```python
from build123d import *

# Parameters (mm, degrees)
EXTRUDE_1_DEPTH     = 4.8
SKETCH_2_W          = 5
SKETCH_2_H          = 4.8
SKETCH_2_W_2        = 2
SKETCH_2_H_2        = 23
EXTRUDE_2_DEPTH     = 12
SKETCH_3_R          = 0.95
CUT_EXTRUDE_1_DEPTH = 5
SKETCH_6_R          = 0.95
CUT_EXTRUDE_4_DEPTH = 32
SKETCH_7_W          = 42.8
SKETCH_7_H          = 6
EXTRUDE_3_DEPTH     = 5
SKETCH_8_W          = 4
SKETCH_8_H          = 32.6
EXTRUDE_4_DEPTH     = 3
SKETCH_9_W          = 42.8
SKETCH_9_H          = 12.6
EXTRUDE_6_DEPTH     = 5
SKETCH_11_R         = 0.95
CUT_EXTRUDE_5_DEPTH = 47.323752007
SKETCH_12_W         = 0.5
SKETCH_12_H         = 25.6
CUT_EXTRUDE_6_DEPTH = 0.5


with BuildPart() as part:
    # 草图1 → 凸台-拉伸1 (new body)
    with BuildSketch(Plane.XY):
        Polygon((12, 0), (28.3, 0), (28.3, -23), (12, -23), (12, -27.8), (4.4, -27.8), (4.4, -23), (0, -23), (0, 0), (4.4, 0), (4.4, 4.8), (12, 4.8), align=None)
    extrude(amount=EXTRUDE_1_DEPTH)

    # 草图2 → 凸台-拉伸2 (add)
    with BuildSketch(Plane.XY.offset(4.8)):
        with Locations((9.5, 2.4)):
            Rectangle(SKETCH_2_W, SKETCH_2_H)
        with Locations((9.5, -25.4)):
            Rectangle(SKETCH_2_W, SKETCH_2_H)
        with Locations((27.3, -11.5)):
            Rectangle(SKETCH_2_W_2, SKETCH_2_H_2)
    extrude(amount=EXTRUDE_2_DEPTH)

    # 草图3 → 切除-拉伸1 (cut)
    with BuildSketch(Plane.ZY.offset(-7)):
        with Locations((10.8, 2.4)):
            Circle(SKETCH_3_R)
        with Locations((10.8, -25.4)):
            Circle(SKETCH_3_R)
    extrude(amount=-CUT_EXTRUDE_1_DEPTH, mode=Mode.SUBTRACT)

    # 草图6 → 切除-拉伸4 (cut)
    with BuildSketch(Plane(origin=(0, 0, 0), x_dir=(1, 0, 0), z_dir=(0, 1, 0))):
        with Locations(Location((14, -2.4, 0), (0, 0, 270))):
            Circle(SKETCH_6_R)
    extrude(amount=-CUT_EXTRUDE_4_DEPTH, mode=Mode.SUBTRACT)

    # 草图7 → 凸台-拉伸3 (add)
    with BuildSketch(Plane(origin=(0, 0, 0), x_dir=(-1, 0, 0), z_dir=(0, 0, -1))):
        with Locations((-6.9, -5.2)):
            Rectangle(SKETCH_7_W, SKETCH_7_H)
    extrude(amount=EXTRUDE_3_DEPTH)

    # 草图8 → 凸台-拉伸4 (add)
    with BuildSketch(Plane.XY):
        with Locations((-2, -11.5)):
            Rectangle(SKETCH_8_W, SKETCH_8_H)
        with Locations((-12.5, -11.5)):
            Rectangle(SKETCH_8_W, SKETCH_8_H)
    extrude(amount=EXTRUDE_4_DEPTH)

    # 草图9 → 凸台-拉伸6 (add)
    with BuildSketch(Plane(origin=(0, 0, 0), x_dir=(-1, 0, 0), z_dir=(0, 0, -1))):
        with Locations((-6.9, -21.5)):
            Rectangle(SKETCH_9_W, SKETCH_9_H)
    extrude(amount=EXTRUDE_6_DEPTH)

    # 草图11 → 切除-拉伸5 (cut, through all)
    with BuildSketch(Plane(origin=(0, 4.8, 0), x_dir=(1, 0, 0), z_dir=(0, 1, 0))):
        with Locations(Location((7, -2.4, 0), (0, 0, 180))):
            Circle(SKETCH_11_R)
    extrude(amount=-CUT_EXTRUDE_5_DEPTH, mode=Mode.SUBTRACT)

    # 草图12 → 切除-拉伸6 (cut)
    with BuildSketch(Plane(origin=(0, 0, -5), x_dir=(-1, 0, 0), z_dir=(0, 0, -1))):
        with Locations((-18.05, -15)):
            Rectangle(SKETCH_12_W, SKETCH_12_H)
        with Locations((-0.75, -15)):
            Rectangle(SKETCH_12_W, SKETCH_12_H)
    extrude(amount=-CUT_EXTRUDE_6_DEPTH, mode=Mode.SUBTRACT)


solid = part.part
```
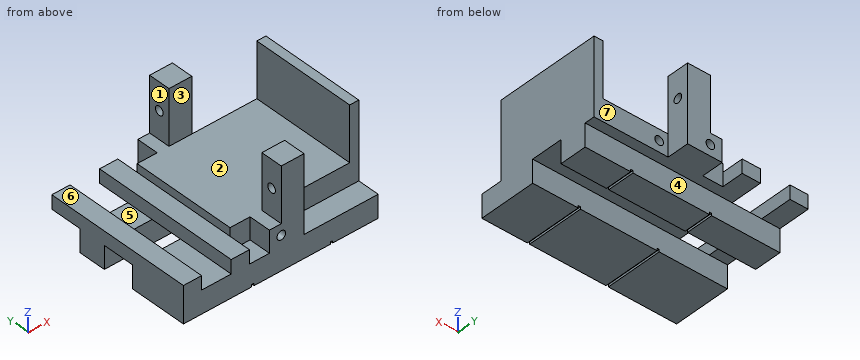
Input: part model. Units: mm. Frame: model coordinates. Face numbers are marked on the shaded views. A direction names the side the tool comes from. Give positions to 0.01 mm unless a question says otherwise; leave off trailing zeros. Write each loop counter-clockwise with the first axis right and the second up, starting at its lowest first coordinate (ties: lowest second). Pieces come first, ordered by that corner, then holes. Notation, with made-up numbers: (54.5, 52.5) - (73.5, 52.5) arc R19 cw to (73.5, 85.5) - close; hole circle Ø9 at (15.25, 44.5). An arc over 180 degrees is marked (long way). Write item = value, one per line. Start each with the question number.
1. Ray query, L1, parallel to Y at x = 9.55, z = 10.8; L2, parallel to Z at x = 7, y = -5; L3, parallel to Z at x = 4, y = -22.5. Return the intervals inside material, ascending.
2. Section query C-C, the plane z = 6.75. Output: boundary loops of the cut face in (x, y), then the cut area to 3 significant figures.
3. First-contact query: pin 1 Ø4 at (x, z) = (15, 1.5) entering from +Y; pin 2 Ø1 at (x, y) = (2, -16.5) entering from +Z; pin 3 Ø2.5 at (y, z) = (3, 9) entering from +X. Flat tips, straight axial feed; report the tip coordinate or a pass-through.
4. Mould query, pull axis Y, two halves, no side actions, for the marked faces 1, 2, 3 and 4. Classes: released by +Y, released by -Y, zero draft, split by the parting line, or undercut.
5. Section query A-A, the plane y = -11. Output: boundary loops of the cut face in (x, z), then the cut area to 3 significant figures.
6. Access query for the marked faces 5, 6 and 7. Directions: +Z, -Z, +X, -X, +Y, -Y. A direction counts if a zero-diameter tool reaches every point of the face in a straight line with its end or side. Return the directions, or none.
7. Section query D-D, the plane y = -25.4. Count the separate pieces of the cut face and the enclosed holes in it, then the cut area to 3 significant figures.
8. Section query B-B, the plane x = 14. Output: boundary loops of the cut face in (y, z).
Check sheet entries:
q1.L1 = -27.8 to -26.35, -24.45 to -23, 0 to 1.45, 3.35 to 4.8
q1.L2 = -5 to 1.45, 3.35 to 4.8
q1.L3 = -5 to 4.8
q2.outline = (7, -27.8) - (12, -27.8) - (12, -23) - (7, -23) - close; (7, 0) - (12, 0) - (12, 4.8) - (7, 4.8) - close; (26.3, -23) - (28.3, -23) - (28.3, 0) - (26.3, 0) - close
q2.area = 94.0 mm2
q3.pin_1 = 0
q3.pin_2 = 4.8
q3.pin_3 = 12
q4.face_1 = zero draft
q4.face_2 = undercut
q4.face_3 = undercut
q4.face_4 = released by +Y
q5.outline = (-14.5, 0) - (-10.5, 0) - (-10.5, 3) - (-14.5, 3) - close; (-4, 0) - (28.3, 0) - (28.3, 16.8) - (26.3, 16.8) - (26.3, 4.8) - (0, 4.8) - (0, 3) - (-4, 3) - close; hole circle Ø1.9 at (7, 2.4); hole circle Ø1.9 at (14, 2.4)
q5.area = 178 mm2
q6.face_5 = +Z, +Y, -Y
q6.face_6 = +Z, -X, +Y, -Y
q6.face_7 = +Z, -Z, +X, +Y
q7.separate_pieces = 2
q7.enclosed_holes = 1
q7.area = 322 mm2
q8.outline = (-27.8, -5) - (-15.2, -5) - (-15.2, 0) - (-8.2, 0) - (-8.2, -5) - (-2.2, -5) - (-2.2, 0) - (0, 0) - (0, 1.45) - (-23, 1.45) - (-23, 0) - (-27.8, 0) - close; (-23, 3.35) - (0, 3.35) - (0, 4.8) - (-23, 4.8) - close
